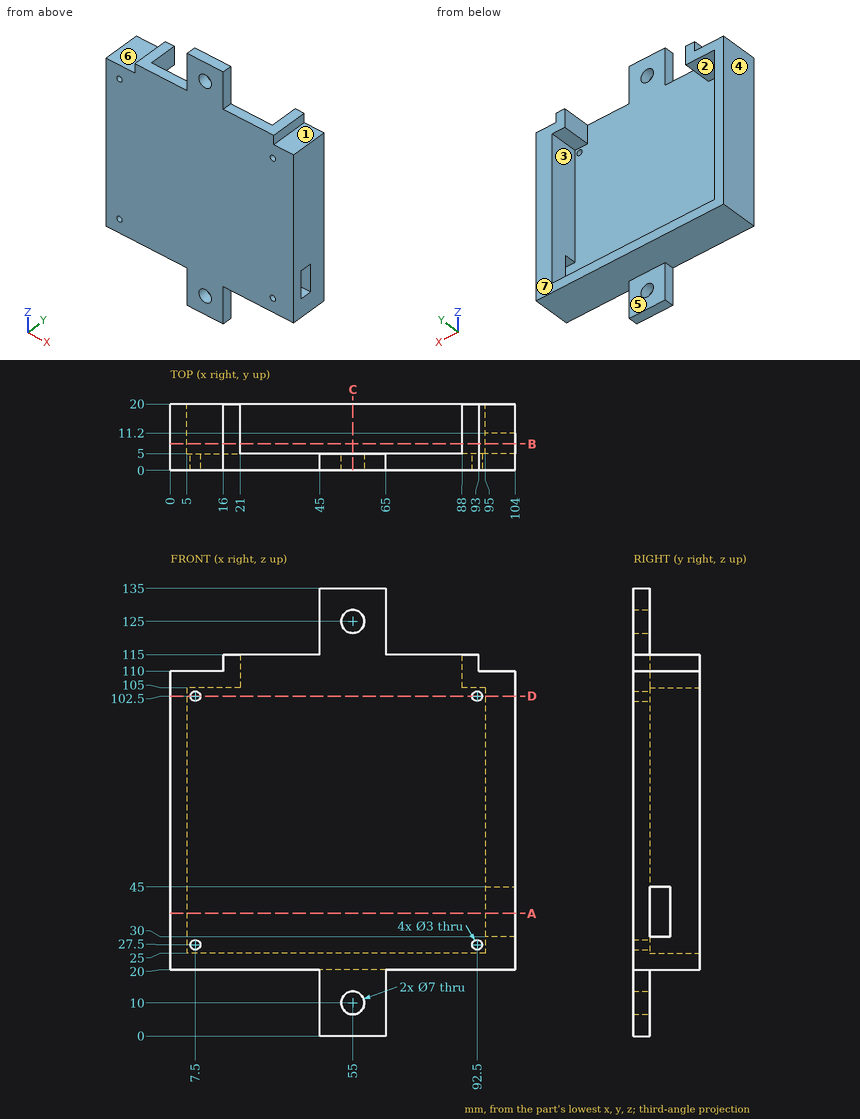
Study the drawing (mm; zero at the part's minimum x, y, z) and answer. A direction names the side the tool comes from. Give positions to 0.01 mm unless a question says otherwise; leave off trailing zeros. Write each loop counter-clockwise with the first axis right and the second up, starting at its lowest first coordinate (ties: lowest second). Pieces come first, ordered by that corner, then holes. Notation, with made-up numbers: (46.5, -27.5) - (51.5, -27.5) arc R22 cw to (51.5, -19.5) - close; hole circle Ø1 at (-10.75, -39.5). An arc over 180 degrees is marked (long way). Use CSV: the item, a comma, the result in double quotes. Start each with the question number.
(1) Find section C-C (x = 55). Give the vertices of the cut face in (y, z), plus the area to 3 significant figures.
(2) Given P1, Ø11, axis at x = 55, z = 125, coming from the +Y side; P2, Ø3, axis at x = 13.5, y = 4.5, coming from the +Z side; P3, Ø2.5, axis at y = 1.5, z = 12, coming from the -X side, each flat-ended and moving along its own axis, determine where each tip first touches the part or whether it passes through.
(3) Find section D-D (z = 102.5). Give the vertices of the cut face in (x, y).
(4) Determine the mould class of the marked faces 1, 2, 3 and 4 for opening direction X: +X half, -X half, draft (parallel to the pull), parting line (faces both ways), or undercut.
(5) Consider line 1 along Z through (x, y) = (7.5, 1.45); line 2 along Z through (x, y) = (92.5, 1); line 3 along X through (y, z) = (3.4, 102.5). Determine where each line is inside the solid, lowest interval first.
(6) For the marked faces 5, 6 and 7, determine the directions among +Z, -Z, +X, -X, +Y, -Y from which every point of the face is accessible in a straight line to the end or side of a thin tool.
(7) Find section A-A (z = 37). Give the vertices of the cut face in (x, y).
(8) Find section B-B (y = 8). Give the vertices of the cut face in (x, z), plus the area to 3 significant figures.
Findings below:
1,outline,"(0, 0) - (5, 0) - (5, 6.5) - (0, 6.5) - close; (0, 13.5) - (5, 13.5) - (5, 20) - (20, 20) - (20, 25) - (5, 25) - (5, 121.5) - (0, 121.5) - close; (0, 128.5) - (5, 128.5) - (5, 135) - (0, 135) - close"
1,area,"680 mm2"
2,P1,"y = 5"
2,P2,"z = 110"
2,P3,"x = 45"
3,outline,"(0, 0) - (6, 0) - (6, 5) - (5, 5) - (5, 20) - (0, 20) - close; (9, 0) - (91, 0) - (91, 5) - (9, 5) - close; (94, 0) - (104, 0) - (104, 20) - (95, 20) - (95, 5) - (94, 5) - close"
4,face 1,"draft"
4,face 2,"undercut"
4,face 3,"undercut"
4,face 4,"-X half"
5,line 1,"20 to 26, 29 to 101, 104 to 110"
5,line 2,"20 to 26, 29 to 101, 104 to 115"
5,line 3,"0 to 6, 9 to 91, 94 to 104"
6,face 5,"-Z, +X, -X, +Y"
6,face 6,"+Z, -X, +Y, -Y"
6,face 7,"+Z, -Z, +X, -X, +Y"
7,outline,"(0, 0) - (104, 0) - (104, 5) - (5, 5) - (5, 20) - (0, 20) - close; (95, 11.2) - (104, 11.2) - (104, 20) - (95, 20) - close"
8,outline,"(0, 20) - (104, 20) - (104, 30) - (95, 30) - (95, 25) - (5, 25) - (5, 105) - (21, 105) - (21, 115) - (16, 115) - (16, 110) - (0, 110) - close; (88, 105) - (95, 105) - (95, 45) - (104, 45) - (104, 110) - (93, 110) - (93, 115) - (88, 115) - close"
8,area,"1,740 mm2"
